from build123d import *

# Parameters (mm, degrees)
F0_R     = 4
F3_R     = 5
F3_R_2   = 4
F7_DEPTH = 15


with BuildPart() as f2:
    # F2: sweep along a path in F1
    with BuildLine(Plane.XZ) as f2_path:
        ThreePointArc((0, 0), (5.0440752924, 2.2394060053), (8, 6.8998935265))
    # F0 (on Right) → F2 (sweep)
    with BuildSketch(Plane.YZ):
        Circle(F0_R)
    sweep(path=f2_path.line)

    # F6: sweep along a path in F5
    with BuildLine(Plane.XZ) as f6_path:
        Line((8, 6.8998935265), (8, 141.8998935265))
    # F3 (on face) → F6 (sweep)
    with BuildSketch(Plane(origin=(3.6385222305, 0, 8.719810755), x_dir=(0.9228788637, 0, -0.3850903828), z_dir=(0.3850903828, 0, 0.9228788637))):
        with Locations((4.7259482702, 0)):
            Circle(F3_R)
        with Locations((4.7259482702, 0)):
            Circle(F3_R_2, mode=Mode.SUBTRACT)
        with Locations((4.7259482702, 0)):
            Circle(F3_R_2)
    sweep(path=f6_path.line)

    # F7 (add): a face of the model
    f7_faces = [f2.faces().sort_by_distance(p)[0] for p in [
        (0, 0, 0),
    ]]
    extrude(f7_faces, amount=F7_DEPTH)


solid = f2.part
Geometry: final body of the model. Coordinates: model frame, mm. A direction names the side the tool comes from. Give positions to 0.01 mm unless a question says otherwise; leave off trailing zeros. Write each loop counter-clockwise with the first axis right and the second up, starting at its lowest first coordinate (ties: lowest second). Pieces come first, ordered by that corner, then holes.
(1) First-contact query: P1, Ø6, axis at y = -3.5, z = 124.5, coming from the +X side; P2, Ø3, axis at y = -2.5, z = 114, coming from the +X side; P3, Ø6, axis at x = -0.5, z = 107.5, coming from the -Y side; P4, Ø5, axis at y = 2.5, z = 49.5, coming from the -X side. Flat tips, straight axial feed; report the tip coordinate or a pass-through.
(2) Cut plane A-A, the plane x = -8. Return loops of the section in (y, z), then the cut area to 3 significant figures.
(3) Access query for faces 1 (the flat face through (7.935, 0.07, 141.927)), 2 (the cylindrical face through (-7.395, -0.867, -3.905)). Directions: +Z, -Z, +X, -X, +Y, -Y. A direction counts if a zero-diameter tool reaches every point of the face in a straight line with its end or side. Return the directions, or none.
(4) Ray query, line 1 (Z direction, x = -2.5, y = -2); line 2 (X direction, y = 4.25, z = 102.5); line 3 (Z direction, x = 3, y = 3.25). Return the intervals inside material, ascending.
Values follow:
1. P1: stops at x = 12.59
1. P2: stops at x = 12.52
1. P3: passes through
1. P4: stops at x = 3.39
2. outline: circle Ø8 at (0, 0)
2. area: 50.3 mm2
3. face 1: +Z, +X, +Y, -Y
3. face 2: -X
4. line 1: z = -3.46 to 3.46
4. line 2: x = 5.57 to 10.43
4. line 3: z = -1.63 to 3.57
